Design review of the part built by this model. Coordinates are the model's own, in mm. Coordinates: 2 decimals unless noted, no trailing zeros. Order: outer loops, then holes, each group sorted by start corner. A loop starts at its lowest first (then second) coordinate and runs counter-clockwise, first axis right, second up. Notation, with made-up numbers: M 75,67 L 83,67 A16 ccw 83,86 Z; hole C -38,-13 d3. An arc over 180 degrees is marked long. Answer in a Markdown table with one row per item.
from build123d import *

# Parameters (mm, degrees)
SKETCH1_R           = 1.905
BOSS_EXTRUDE1_DEPTH = 1.5748


with BuildPart() as part:
    # Sketch1 → Boss-Extrude1 (new body)
    with BuildSketch(Plane(origin=(0, 0, 0), x_dir=(1, 0, 0), z_dir=(0, 1, 0))):
        with BuildLine():
            Line((-25.658087094, 37.465), (25.658087094, 37.465))
            ThreePointArc((25.658087094, 37.465), (32.108905761, 32.108905761), (37.465, 25.658087094))
            Line((37.465, 25.658087094), (37.465, -25.658087094))
            ThreePointArc((37.465, -25.658087094), (32.108905761, -32.108905761), (25.658087094, -37.465))
            Line((25.658087094, -37.465), (9.48055, -37.465))
            Line((9.48055, -37.465), (9.48055, -34.925))
            ThreePointArc((9.48055, -34.925), (0, -25.44445), (-9.48055, -34.925))
            Line((-9.48055, -34.925), (-9.48055, -37.465))
            Line((-9.48055, -37.465), (-25.658087094, -37.465))
            ThreePointArc((-25.658087094, -37.465), (-32.108905761, -32.108905761), (-37.465, -25.658087094))
            Line((-37.465, -25.658087094), (-37.465, 25.658087094))
            ThreePointArc((-37.465, 25.658087094), (-32.108905761, 32.108905761), (-25.658087094, 37.465))
        make_face()
        with Locations(Location((13.8176, -7.97759508, 0), (0, 0, 270))):
            Circle(SKETCH1_R, mode=Mode.SUBTRACT)
        with Locations(Location((0, 15.955190159, 0), (0, 0, 270))):
            Circle(SKETCH1_R, mode=Mode.SUBTRACT)
        with Locations(Location((-13.8176, -7.97759508, 0), (0, 0, 270))):
            Circle(SKETCH1_R, mode=Mode.SUBTRACT)
        with Locations(Location((-19.4945, -2.286, 0), (0, 0, 270))):
            Circle(SKETCH1_R, mode=Mode.SUBTRACT)
        with Locations(Location((19.4945, -2.286, 0), (0, 0, 270))):
            Circle(SKETCH1_R, mode=Mode.SUBTRACT)
    extrude(amount=BOSS_EXTRUDE1_DEPTH)


solid = part.part
(1) Draft analysis for pull direction X (two halves, no side actions). For faces 1 (the cylindrical face through (0.08, 0.78, -17.86)), 2 (the cylindrical face through (-32.03, 0.78, 32.19)), 3 (the cylindrical face through (32.03, 0.78, -32.19)), state which applies: pulls with the +X half, pulls with the -X half, needs draft (parallel to the pull), parting line crosses it, or undercut.
Return value:
| item | result |
|---|---|
| face 1 | undercut |
| face 2 | pulls with the -X half |
| face 3 | pulls with the +X half |
(2) Add section C-C, the plane z = -16.5. Give the boundary of the cut face in (x, y) (3 decimals).
Return value:
| item | result |
|---|---|
| outline | M -37.465,0 L -1.825,0 L -1.825,1.575 L -37.465,1.575 Z; M 1.825,0 L 37.465,0 L 37.465,1.575 L 1.825,1.575 Z |
(3) Insertion check: pin 1 Ø0.8 at (y, z) = (0.5, 36) entering from -X; pin 2 Ø3 at (x, z) = (-13.82, 7.98) entering from -Y. Each pin has a flat end and moves straight along its axis. Give the tip position at first contact, or say it passes through.
Return value:
| item | result |
|---|---|
| pin 1 | stops at x = -28.19 |
| pin 2 | passes through |
(4) Add section A-A, the plane x = 0. Give the boundary of the cut face in (y, z) (3 decimals), and give its area (3 significant figures).
Return value:
| item | result |
|---|---|
| outline | M 0,-37.465 L 1.575,-37.465 L 1.575,-17.86 L 0,-17.86 Z; M 0,-14.05 L 1.575,-14.05 L 1.575,25.444 L 0,25.444 Z |
| area | 93.1 mm2 |
(5) Add section B-B, the plane y = 0.4. Give the boundary of the cut face in (x, z) (1 decimal).
Return value:
| item | result |
|---|---|
| outline | M -37.5,-25.7 A45.4 ccw -25.7,-37.5 L 25.7,-37.5 A45.4 ccw 37.5,-25.7 L 37.5,25.7 A45.4 ccw 25.7,37.5 L 9.5,37.5 L 9.5,34.9 A9.5 cw -9.5,34.9 L -9.5,37.5 L -25.7,37.5 A45.4 ccw -37.5,25.7 Z; hole C -19.5,2.3 d3.8; hole C -13.8,8 d3.8; hole C 0,-16 d3.8; hole C 13.8,8 d3.8; hole C 19.5,2.3 d3.8 |
(6) For line 1 along X through (y, z) = (0.9, 28.5); line 2 along X through (y, z) = (1.4, 29); line 3 along Z through (x, y) = (19, 0.95) (3 decimals), list the stretches that pass through material, from the lowest coordinate up. Write a range as from..to.
Return value:
| item | result |
|---|---|
| line 1 | x = -35.35..-6.97, 6.97..35.35 |
| line 2 | x = -34.94..-7.4, 7.4..34.94 |
| line 3 | z = -37.465..0.446, 4.126..37.465 |
